from build123d import *

# Parameters (mm, degrees)
SKETCH1_R            = 1.6
BOSS_EXTRUDE1_DEPTH  = 2
FILLET1_R            = 10
SKETCH2_R            = 4
BOSS_EXTRUDE3_DEPTH  = 2
SKETCH4_R            = 1.6
CUT_EXTRUDE2_DEPTH   = 4
CUT_EXTRUDE3_DEPTH   = 10
SKETCH6_R            = 3
SKETCH6_R_2          = 1.6
BOSS_EXTRUDE4_DEPTH  = 2
SKETCH7_R            = 1.6
CUT_EXTRUDE4_DEPTH   = 10
SKETCH8_W            = 36
SKETCH8_H            = 10
CUT_EXTRUDE6_DEPTH   = 9.5
FILLET3_R            = 3
SKETCH9_R            = 1.6
BOSS_EXTRUDE5_DEPTH  = 2
SKETCH10_R           = 1.6
BOSS_EXTRUDE6_DEPTH  = 2
SKETCH11_R           = 1.6
CUT_EXTRUDE7_DEPTH   = 10
BOSS_EXTRUDE7_DEPTH  = 2
SKETCH13_R           = 1.6
CUT_EXTRUDE9_DEPTH   = 5.5
BOSS_EXTRUDE8_DEPTH  = 2
SKETCH16_R           = 1.6
CUT_EXTRUDE10_DEPTH  = 10
SKETCH17_R           = 2.884899687
BOSS_EXTRUDE9_DEPTH  = 1
SKETCH18_R           = 1.6
BOSS_EXTRUDE10_DEPTH = 3
SKETCH19_R           = 1.6
SKETCH19_R_2         = 1.5
CUT_EXTRUDE11_DEPTH  = 2
SKETCH20_R           = 1.6
CUT_EXTRUDE12_DEPTH  = 10
SKETCH21_R           = 1.5
CUT_EXTRUDE13_DEPTH  = 8.5


with BuildPart() as part:
    # Sketch1 → Boss-Extrude1 (new body)
    with BuildSketch(Plane(origin=(0, 0, 0), x_dir=(1, 0, 0), z_dir=(0, 1, 0))):
        with BuildLine():
            Line((-4, -45), (-4, -30))
            Line((-4, -30), (-4, -19))
            Line((-4, -19), (-22, -19))
            ThreePointArc((-22, -19), (-24.828427125, -17.828427125), (-26, -15))
            Line((-26, -15), (-26, -5))
            ThreePointArc((-26, -5), (-24.828427125, -2.171572875), (-22, -1))
            Line((-22, -1), (-4, -1))
            Line((-4, -1), (-4, 0))
            ThreePointArc((-4, 0), (0, 4), (4, 0))
            Line((4, 0), (4, -1))
            Line((4, -1), (22, -1))
            ThreePointArc((22, -1), (24.828427125, -2.171572875), (26, -5))
            Line((26, -5), (26, -15))
            ThreePointArc((26, -15), (24.828427125, -17.828427125), (22, -19))
            Line((22, -19), (4, -19))
            Line((4, -19), (4, -30))
            Line((4, -30), (4, -45))
            ThreePointArc((4, -45), (0, -49), (-4, -45))
        make_face()
        with Locations((-22, -5)):
            Circle(SKETCH1_R, mode=Mode.SUBTRACT)
        Circle(SKETCH1_R, mode=Mode.SUBTRACT)
        with Locations((22, -5)):
            Circle(SKETCH1_R, mode=Mode.SUBTRACT)
        with Locations((22, -15)):
            Circle(SKETCH1_R, mode=Mode.SUBTRACT)
        with Locations((-22, -15)):
            Circle(SKETCH1_R, mode=Mode.SUBTRACT)
        with BuildLine():
            ThreePointArc((-1.6, -45), (0, -46.6), (1.6, -45))
            Line((1.6, -45), (1.6, -30))
            ThreePointArc((1.6, -30), (0, -28.4), (-1.6, -30))
            Line((-1.6, -30), (-1.6, -45))
        make_face(mode=Mode.SUBTRACT)
    extrude(amount=BOSS_EXTRUDE1_DEPTH)

    # Fillet1
    fillet1_edges = [part.edges().sort_by_distance(p)[0] for p in [
        (-4, 1, 19),
        (4, 1, 19),
    ]]
    fillet(fillet1_edges, radius=FILLET1_R)

    # Sketch2 → Boss-Extrude3 (add)
    with BuildSketch(Plane(origin=(0, 2, 0), x_dir=(1, 0, 0), z_dir=(0, 1, 0))):
        with BuildLine():
            ThreePointArc((-3.708099244, 1.5), (-2.797344782, 2.859171588), (-1.41859085, 3.74))
            ThreePointArc((-1.41859085, 3.74), (0, 4.6), (1.41859085, 3.74))
            ThreePointArc((1.41859085, 3.74), (2.797344782, 2.859171588), (3.708099244, 1.5))
            ThreePointArc((3.708099244, 1.5), (3.92634671, 2.23593095), (4, 3))
            ThreePointArc((4, 3), (0, 7), (-4, 3))
            ThreePointArc((-4, 3), (-3.92634671, 2.23593095), (-3.708099244, 1.5))
        make_face()
        with BuildLine():
            ThreePointArc((4, 3), (3.92634671, 2.23593095), (3.708099244, 1.5))
            ThreePointArc((3.708099244, 1.5), (3.92634671, 0.76406905), (4, 0))
            Line((4, 0), (4, 3))
        make_face()
        with BuildLine():
            ThreePointArc((-4, 0), (-3.92634671, 0.76406905), (-3.708099244, 1.5))
            ThreePointArc((-3.708099244, 1.5), (-3.92634671, 2.23593095), (-4, 3))
            Line((-4, 3), (-4, 0))
        make_face()
        Circle(SKETCH2_R)
    extrude(amount=-BOSS_EXTRUDE3_DEPTH)

    # Sketch4 → Cut-Extrude2 (cut)
    with BuildSketch(Plane(origin=(0, 2, 0), x_dir=(1, 0, 0), z_dir=(0, 1, 0))):
        with Locations((0, 3)):
            Circle(SKETCH4_R)
    extrude(amount=-CUT_EXTRUDE2_DEPTH, mode=Mode.SUBTRACT)

    # Sketch5 → Cut-Extrude3 (cut)
    with BuildSketch(Plane(origin=(0, 2, 0), x_dir=(1, 0, 0), z_dir=(0, 1, 0))):
        Polygon((-4, -1), (4, -1), (9.121752044, 12.8952039), (-11.957584595, 14.407484274), align=None)
    extrude(amount=-CUT_EXTRUDE3_DEPTH, mode=Mode.SUBTRACT)

    # Sketch6 → Boss-Extrude4 (add)
    with BuildSketch(Plane(origin=(0, 2, 0), x_dir=(1, 0, 0), z_dir=(0, 1, 0))):
        with Locations((0, -1)):
            Circle(SKETCH6_R)
        with Locations((0, -1)):
            Circle(SKETCH6_R_2, mode=Mode.SUBTRACT)
    extrude(amount=-BOSS_EXTRUDE4_DEPTH)

    # Sketch7 → Cut-Extrude4 (cut)
    with BuildSketch(Plane(origin=(0, 2, 0), x_dir=(1, 0, 0), z_dir=(0, 1, 0))):
        with Locations((0, -1)):
            Circle(SKETCH7_R)
    extrude(amount=-CUT_EXTRUDE4_DEPTH, mode=Mode.SUBTRACT)

    # Sketch8 → Cut-Extrude6 (cut)
    with BuildSketch(Plane(origin=(0, 2, 0), x_dir=(1, 0, 0), z_dir=(0, 1, 0))):
        with Locations((0, -10)):
            Rectangle(SKETCH8_W, SKETCH8_H)
    extrude(amount=-CUT_EXTRUDE6_DEPTH, mode=Mode.SUBTRACT)

    # Fillet3
    fillet3_edges = [part.edges().sort_by_distance(p)[0] for p in [
        (-18, 1, 5),
        (18, 1, 5),
        (18, 1, 15),
        (-18, 1, 15),
    ]]
    fillet(fillet3_edges, radius=FILLET3_R)

    # Sketch9 → Boss-Extrude5 (add)
    with BuildSketch(Plane(origin=(0, 2, 0), x_dir=(1, 0, 0), z_dir=(0, 1, 0))):
        with Locations((0, -1)):
            Circle(SKETCH9_R)
    extrude(amount=-BOSS_EXTRUDE5_DEPTH)

    # Sketch10 → Boss-Extrude6 (add)
    with BuildSketch(Plane(origin=(0, 2, 0), x_dir=(1, 0, 0), z_dir=(0, 1, 0))):
        with BuildLine():
            Line((3, -1), (3, 3))
            ThreePointArc((3, 3), (0, 6), (-3, 3))
            Line((-3, 3), (-3, -1))
            Line((-3, -1), (3, -1))
        make_face()
        with Locations((0, 3)):
            Circle(SKETCH10_R, mode=Mode.SUBTRACT)
    extrude(amount=-BOSS_EXTRUDE6_DEPTH)

    # Sketch11 → Cut-Extrude7 (cut)
    with BuildSketch(Plane(origin=(0, 2, 0), x_dir=(1, 0, 0), z_dir=(0, 1, 0))):
        with Locations((0, 3)):
            Circle(SKETCH11_R)
    extrude(amount=-CUT_EXTRUDE7_DEPTH, mode=Mode.SUBTRACT)

    # Sketch12 → Boss-Extrude7 (add)
    with BuildSketch(Plane(origin=(0, 2, 0), x_dir=(1, 0, 0), z_dir=(0, 1, 0))):
        with BuildLine():
            Line((-3, 3), (-3, 4))
            ThreePointArc((-3, 4), (0, 7), (3, 4))
            Line((3, 4), (3, 3))
            Line((3, 3), (2.828427125, 3))
            ThreePointArc((2.828427125, 3), (0, 1), (-2.828427125, 3))
            Line((-2.828427125, 3), (-3, 3))
        make_face()
    extrude(amount=-BOSS_EXTRUDE7_DEPTH)

    # Sketch13 → Cut-Extrude9 (cut)
    with BuildSketch(Plane(origin=(0, 2, 0), x_dir=(1, 0, 0), z_dir=(0, 1, 0))):
        with Locations((0, 4)):
            Circle(SKETCH13_R)
    extrude(amount=-CUT_EXTRUDE9_DEPTH, mode=Mode.SUBTRACT)

    # Sketch15 → Boss-Extrude8 (add)
    with BuildSketch(Plane(origin=(0, 2, 0), x_dir=(1, 0, 0), z_dir=(0, 1, 0))):
        with BuildLine():
            Line((-4, -45), (-4, -23.953750057))
            Line((-4, -23.953750057), (4, -23.953750057))
            Line((4, -23.953750057), (4, -45))
            ThreePointArc((4, -45), (0, -49), (-4, -45))
        make_face()
    extrude(amount=-BOSS_EXTRUDE8_DEPTH)

    # Sketch16 → Cut-Extrude10 (cut)
    with BuildSketch(Plane(origin=(0, 2, 0), x_dir=(1, 0, 0), z_dir=(0, 1, 0))):
        with Locations((0, -45)):
            Circle(SKETCH16_R)
        with Locations((0, -36)):
            Circle(SKETCH16_R)
    extrude(amount=-CUT_EXTRUDE10_DEPTH, mode=Mode.SUBTRACT)

    # Sketch17 → Boss-Extrude9 (add)
    with BuildSketch(Plane(origin=(0, 2, 0), x_dir=(1, 0, 0), z_dir=(0, 1, 0))):
        with Locations((0, -36)):
            Circle(SKETCH17_R)
    extrude(amount=-BOSS_EXTRUDE9_DEPTH)

    # Sketch18 → Boss-Extrude10 (add)
    with BuildSketch(Plane(origin=(0, 1, 0), x_dir=(-1, 0, 0), z_dir=(0, -1, 0))):
        with Locations((0, -36)):
            Circle(SKETCH18_R)
    extrude(amount=BOSS_EXTRUDE10_DEPTH)

    # Sketch19 → Cut-Extrude11 (cut)
    with BuildSketch(Plane(origin=(0, -2, 0), x_dir=(-1, 0, 0), z_dir=(0, -1, 0))):
        with Locations((0, -36)):
            Circle(SKETCH19_R)
        with Locations((0, -36)):
            Circle(SKETCH19_R_2, mode=Mode.SUBTRACT)
    extrude(amount=-CUT_EXTRUDE11_DEPTH, mode=Mode.SUBTRACT)

    # Sketch20 → Cut-Extrude12 (cut)
    with BuildSketch(Plane(origin=(0, 0, 0), x_dir=(-1, 0, 0), z_dir=(0, -1, 0))):
        with Locations((0, -40.5)):
            Circle(SKETCH20_R)
    extrude(amount=-CUT_EXTRUDE12_DEPTH, mode=Mode.SUBTRACT)

    # Sketch21 → Cut-Extrude13 (cut)
    with BuildSketch(Plane(origin=(0, 0, 0), x_dir=(-1, 0, 0), z_dir=(0, -1, 0))):
        with Locations((0, -36)):
            Circle(SKETCH21_R)
    extrude(amount=CUT_EXTRUDE13_DEPTH, mode=Mode.SUBTRACT)


solid = part.part
Here's how the part is built. I have some questions about the finished solid (model axes, mm). A direction names the side the tool comes from. Coordinates: 2 decimals unless noted, no trailing zeros. Loops run counter-clockwise (first coordinate to the right, second up) from the corner with the lowest first, then second, coordinate; pieces in that order, holes last.
1. Imagine slicing it at D-D, the plane x = 16.5. Please give me the cut outline in (y, z), and give its area (3 significant figures).
2. For faces 4 (the flat face through (-18, 1, 19)), 5 (the flat face through (0, 1, 15)), 6 (the flat face through (12, 1, 1)), which set-ups out of +Z, -Z, +X, -X, +Y, -Y let a thin tool reach every point of the face, with its end or its side?
3. Imagine slicing it at A-A, the plane z = 40.5. Please give me the cut outline in (x, y).
4. Imagine slicing it at B-B, the plane x = 0. Please give me the cut outline in (y, z), and give its area (3 significant figures).
5. I need wall thicknesses on L1, parallel to Z at x = 0, y = 1.4; L2, parallel to Z at x = -22, y = 0.5; L3, parallel to X at y = 0.75, z = -4. Which ranges of each line are inside material? Lowest first, please.
6. If we mould it in two halves opening along X, with no side actions, what happens to faces 1 (the flat face through (-13, 1, 1)), 2 (the cylindrical face through (17.14, 0.99, 5.9)), 3 (the cylindrical face through (6.85, 1.01, 22.01))? For each: pulls with the +X half, pulls with the -X half, needs draft (parallel to the pull), parting line crosses it, or undercut.
7. For P1, Ø1, axis at y = 0.5, z = 38, coming from the -X side; P2, Ø1, axis at x = -19.5, y = 0.5, coming from the +Z side; P3, Ø0.6, axis at y = 1.5, z = -1.5, coming from the +X side, each with a flat end and sliding along its axis, tell me the tip position at first contact or that it passes through.
8. Imagine slicing it at C-C, the plane y = 1.2. Count the separate pieces of the cut face and the enclosed holes in it, and give its area (3 significant figures).
Taken from the geometry:
1. outline: (0, 1) - (2, 1) - (2, 5.4) - (0, 5.4) - close; (0, 14.6) - (2, 14.6) - (2, 19) - (0, 19) - close
1. area: 17.6 mm2
2. face 4: +Z, -X, +Y, -Y
2. face 5: +Y, -Y
2. face 6: -Z, +X, +Y, -Y
3. outline: (-4, 0) - (-1.6, 0) - (-1.6, 2) - (-4, 2) - close; (1.6, 0) - (4, 0) - (4, 2) - (1.6, 2) - close
4. outline: (0, -7) - (2, -7) - (2, -5.6) - (0, -5.6) - close; (0, -2.4) - (2, -2.4) - (2, 5) - (0, 5) - close; (0, 15) - (2, 15) - (2, 38.9) - (0, 38.9) - close; (0, 42.1) - (2, 42.1) - (2, 43.4) - (0, 43.4) - close; (0, 46.6) - (2, 46.6) - (2, 49) - (0, 49) - close
4. area: 72.8 mm2
5. L1: z = -7 to -5.6, -2.4 to 5, 15 to 38.9, 42.1 to 43.4, 46.6 to 49
5. L2: z = 1 to 3.4, 6.6 to 13.4, 16.6 to 19
5. L3: x = -3 to -1.6, 1.6 to 3
6. face 1: needs draft
6. face 2: undercut
6. face 3: pulls with the +X half
7. P1: stops at x = -4
7. P2: stops at z = 19
7. P3: stops at x = 3
8. separate pieces: 1
8. enclosed holes: 8
8. area: 834 mm2
